```python
from build123d import *

# Parameters (mm, degrees)
SKETCH1_W           = 65
SKETCH1_H           = 6
BOSS_EXTRUDE1_DEPTH = 2
SKETCH2_R           = 1.2
CUT_EXTRUDE1_DEPTH  = 66.306967469
SKETCH3_W           = 52
SKETCH3_H           = 1.2
BOSS_EXTRUDE2_DEPTH = 2
FILLET1_R           = 1.2
FILLET3_R           = 1
FILLET4_R           = 1
FILLET5_R           = 1
SKETCH4_R           = 2.15
SKETCH4_R_2         = 1.55
CUT_EXTRUDE2_DEPTH  = 0.8


with BuildPart() as part:
    # Sketch1 → Boss-Extrude1 (new body)
    with BuildSketch(Plane(origin=(0, 0, 0), x_dir=(1, 0, 0), z_dir=(0, 1, 0))):
        with Locations((32.5, -3)):
            Rectangle(SKETCH1_W, SKETCH1_H)
    extrude(amount=BOSS_EXTRUDE1_DEPTH)

    # Sketch2 → Cut-Extrude1 (cut, through all)
    with BuildSketch(Plane(origin=(0, 2, 0), x_dir=(1, 0, 0), z_dir=(0, 1, 0))):
        with Locations(Location((62, -3, 0), (0, 0, 270))):
            Circle(SKETCH2_R)
        with Locations(Location((3, -3, 0), (0, 0, 270))):
            Circle(SKETCH2_R)
    extrude(amount=-CUT_EXTRUDE1_DEPTH, mode=Mode.SUBTRACT)

    # Sketch3 → Boss-Extrude2 (add)
    with BuildSketch(Plane(origin=(0, 2, 0), x_dir=(1, 0, 0), z_dir=(0, 1, 0))):
        with Locations((32.5, -3)):
            Rectangle(SKETCH3_W, SKETCH3_H)
    extrude(amount=BOSS_EXTRUDE2_DEPTH)

    # Fillet1
    fillet1_edges = [part.edges().sort_by_distance(p)[0] for p in [
        (0, 1, 0),
        (65, 1, 0),
        (65, 1, 6),
        (0, 1, 6),
    ]]
    fillet(fillet1_edges, radius=FILLET1_R)

    # Fillet3
    fillet3_edges = [part.edges().sort_by_distance(p)[0] for p in [
        (6.5, 4, 3),
        (58.5, 4, 3),
    ]]
    fillet(fillet3_edges, radius=FILLET3_R)

    # Fillet4
    fillet4_edges = [part.edges().sort_by_distance(p)[0] for p in [
        (32.5, 2, 3.6),
        (32.5, 2, 2.4),
    ]]
    fillet(fillet4_edges, radius=FILLET4_R)

    # Fillet5
    fillet5_edges = [part.edges().sort_by_distance(p)[0] for p in [
        (58.5, 2, 3),
        (6.5, 2, 3),
    ]]
    fillet(fillet5_edges, radius=FILLET5_R - 0.0001)  # a hair under: the kernel refuses the full size

    # Sketch4 → Cut-Extrude2 (cut)
    # profile 1 of 2: a face of its own
    with BuildSketch(Plane(origin=(0, 0, 0), x_dir=(-1, 0, 0), z_dir=(0, -1, 0))):
        with Locations(Location((-20, -3, 0), (0, 0, 90))):
            Circle(SKETCH4_R)
        with Locations(Location((-20, -3, 0), (0, 0, 90))):
            Circle(SKETCH4_R_2, mode=Mode.SUBTRACT)
    # profile 2 of 2: a face of its own
    with BuildSketch(Plane(origin=(0, 0, 0), x_dir=(-1, 0, 0), z_dir=(0, -1, 0))):
        with Locations(Location((-45, -3, 0), (0, 0, 90))):
            Circle(SKETCH4_R)
        with Locations(Location((-45, -3, 0), (0, 0, 90))):
            Circle(SKETCH4_R_2, mode=Mode.SUBTRACT)
    extrude(amount=-CUT_EXTRUDE2_DEPTH, mode=Mode.SUBTRACT)


solid = part.part
```
Read the model definition and answer for the solid it produces. Units are mm, in the model's axes. A direction names the side the tool comes from. Give positions to 0.01 mm unless a question says otherwise; leave off trailing zeros. Loops run counter-clockwise (first coordinate to the right, second up) from the corner with the lowest first, then second, coordinate; pieces in that order, holes last.
Item 1: The mould has two halves that part along X. Classify faces 4 (the flat face through (0, 1, 3)), 5 (the cylindrical face through (17.9, 0.39, 3.47)), 6 (the flat face through (45, 0, 3)), 7 (the cylindrical face through (58.9, 2.2, 3)): released by +X, released by -X, zero draft, split by the parting line, or undercut.
Item 2: Find the intervals of material crossed by line 1 along X through (y, z) = (1.9, 3); line 2 along X through (y, z) = (1.5, 3.5); line 3 along Y through (x, z) = (20, 1.25), in increasing order.
Item 3: The part is cut by section B-B (y = 1.35). Write down the section's boundary in (x, z).
Item 4: The part is cut by section C-C (x = 40.5). Write down the section's boundary in (y, z), and give its area (3 significant figures).
Item 5: For faces 1 (the flat face through (32.1, 3.5, 3.6)), 2 (the flat face through (32.1, 3.5, 2.4)), 3 (the cylindrical face through (47.13, 0.39, 3.28)), determine the directions among +Z, -Z, +X, -X, +Y, -Y from which every point of the face is accessible in a straight line to the end or side of a thin tool.
Item 6: Each of these flat-tipped pins is pushed along its axis until it touches: pin 1 Ø3.5 at (x, z) = (21, 3) entering from -Y; pin 2 Ø0.5 at (x, y) = (27, 3.5) entering from -Z. Where does it stop, or does it pass through?
Item 7: The part is cut by section A-A (x = 62). Write down the section's boundary in (y, z).
Item 8: The part is cut by section D-D (z = 3). Give the number of separate pieces and of enclosed holes in the cut face, and give its area (3 significant figures).
Taken from the geometry:
1. face 4: released by -X
1. face 5: undercut
1. face 6: zero draft
1. face 7: released by +X
2. line 1: x = 0 to 1.8, 4.2 to 60.8, 63.2 to 65
2. line 2: x = 0 to 1.91, 4.09 to 60.91, 63.09 to 65
2. line 3: y = 0.8 to 2
3. outline: (0, 1.2) arc R1.2 ccw to (1.2, 0) - (63.8, 0) arc R1.2 ccw to (65, 1.2) - (65, 4.8) arc R1.2 ccw to (63.8, 6) - (1.2, 6) arc R1.2 ccw to (0, 4.8) - close; hole circle Ø2.4 at (3, 3); hole circle Ø2.4 at (62, 3)
4. outline: (0, 0) - (2, 0) - (2, 1.4) arc R1 cw to (3, 2.4) - (4, 2.4) - (4, 3.6) - (3, 3.6) arc R1 cw to (2, 4.6) - (2, 6) - (0, 6) - close
4. area: 14.8 mm2
5. face 1: +Z, +X, -X, +Y
5. face 2: -Z, +X, -X, +Y
5. face 3: -Y
6. pin 1: stops at y = 0
6. pin 2: stops at z = 2.4
7. outline: (0, 0) - (2, 0) - (2, 1.8) - (0, 1.8) - close; (0, 4.2) - (2, 4.2) - (2, 6) - (0, 6) - close
8. separate pieces: 3
8. enclosed holes: 0
8. area: 222 mm2
